Here's the drawing with two shaded views (mm, measured from the low corner). I have some questions. Give positions to 0.01 mm unless a question says otherwise; leave off trailing zeros. Loops run counter-clockwise (first coordinate to the right, second up) from the corner with the lowest first, then second, coordinate; pieces in that order, holes last. Notation, with made-up numbers: (41.5, -21.75) -> (78.5, -21.75) arc R20 cw to (78.5, -10.75) -> close; hole circle Ø1 at (-26, 87). An arc over 180 degrees is marked (long way). Answer in a Markdown table with one row per item. Add a question column.
Item 1: If we section it at A-A (y = 10): Write out the boundary of the cut face in (x, z).
Item 2: If I drill on line 1 (Y direction, x = 10, z = 0.45); line 2 (X direction, y = 80, z = 1.1); line 3 (Y direction, x = 9, z = 0.1), over which ranges is the centre line in solid material (lowest first)?
Item 3: If we section it at B-B (x = 70): Write out the boundary of the cut face in (y, z).
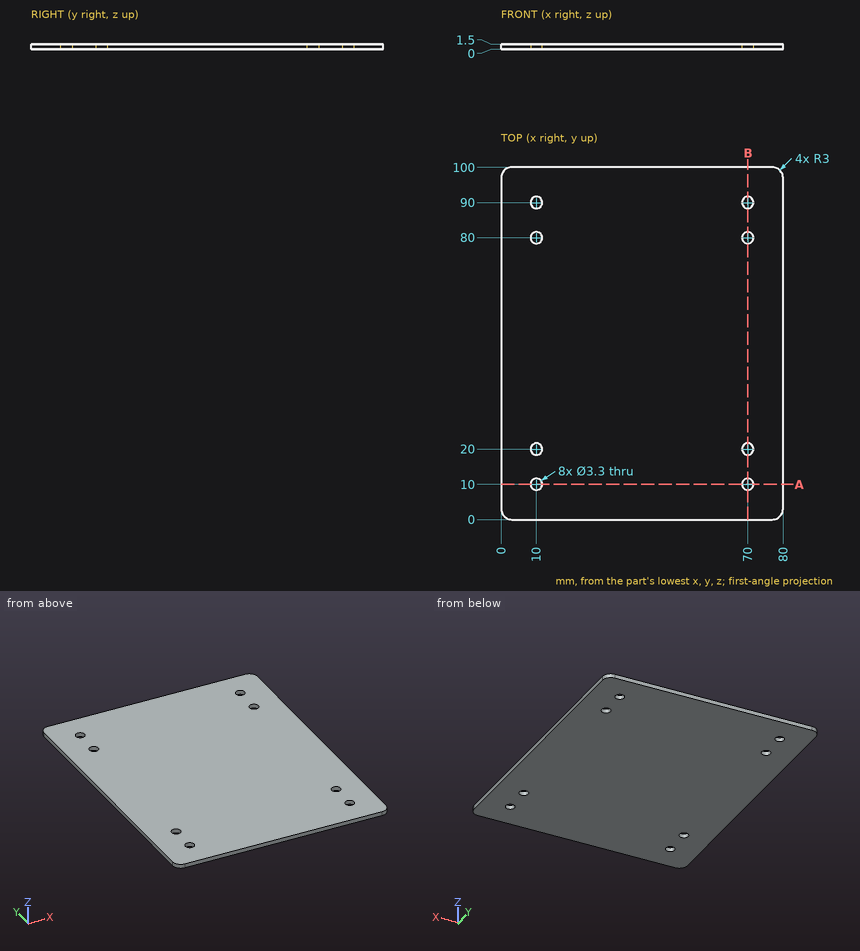
Recorded:
| question | item | result |
|---|---|---|
| 1 | outline | (0, 0) -> (8.35, 0) -> (8.35, 1.5) -> (0, 1.5) -> close; (11.65, 0) -> (68.35, 0) -> (68.35, 1.5) -> (11.65, 1.5) -> close; (71.65, 0) -> (80, 0) -> (80, 1.5) -> (71.65, 1.5) -> close |
| 2 | line 1 | y = 0 to 8.35, 11.65 to 18.35, 21.65 to 78.35, 81.65 to 88.35, 91.65 to 100 |
| 2 | line 2 | x = 0 to 8.35, 11.65 to 68.35, 71.65 to 80 |
| 2 | line 3 | y = 0 to 8.69, 11.31 to 18.69, 21.31 to 78.69, 81.31 to 88.69, 91.31 to 100 |
| 3 | outline | (0, 0) -> (8.35, 0) -> (8.35, 1.5) -> (0, 1.5) -> close; (11.65, 0) -> (18.35, 0) -> (18.35, 1.5) -> (11.65, 1.5) -> close; (21.65, 0) -> (78.35, 0) -> (78.35, 1.5) -> (21.65, 1.5) -> close; (81.65, 0) -> (88.35, 0) -> (88.35, 1.5) -> (81.65, 1.5) -> close; (91.65, 0) -> (100, 0) -> (100, 1.5) -> (91.65, 1.5) -> close |
